The model under review builds one solid part; all positions refer to its coordinate system, in mm. A direction names the side the tool comes from. Coordinates: 2 decimals unless noted, no trailing zeros. Write each loop counter-clockwise with the first axis right and the second up, starting at its lowest first coordinate (ties: lowest second). Pieces come first, ordered by that corner, then holes. Notation, with made-up numbers: M 84,-39.5 L 102,-39.5 A17 cw 102,-20.5 Z; hole C 23,-36 d1. An arc over 180 degrees is marked long. Answer as CSV lines item,"result". Start each with the question number.
from build123d import *
from OCP.BRepFilletAPI import BRepFilletAPI_MakeChamfer

# Parameters (mm, degrees)
SKETCH_1_W          = 44.524667954
SKETCH_1_H          = 33.301696974
EXTRUDE_1_DEPTH     = 25
SKETCH_2_W          = 25
SKETCH_2_H          = 44.524667954
EXTRUDE_2_DEPTH     = 20
SKETCH_3_R          = 4
CUT_EXTRUDE_1_DEPTH = 67.802936569
SKETCH_4_W          = 57.585084074
SKETCH_4_H          = 20.16053609
CUT_EXTRUDE_2_DEPTH = 23
CHAMFER_2_SIZE      = 10
CHAMFER_2_SIZE2     = 6.494075932
SKETCH_5_W          = 25
SKETCH_5_H          = 60
EXTRUDE_3_DEPTH     = 12
FILLET_2_R          = 7
SKETCH_6_R          = 12.5
CUT_EXTRUDE_3_DEPTH = 59.13936943


with BuildPart() as part:
    # Эскиз1 → Вытянуть1 (new body)
    with BuildSketch(Plane(origin=(0, 0, 0), x_dir=(0, 0, -1), z_dir=(1, 0, 0))):
        with Locations((0, 6.421024908)):
            Rectangle(SKETCH_1_W, SKETCH_1_H)
    extrude(amount=EXTRUDE_1_DEPTH)

    # Эскиз2 → Вытянуть2 (add)
    with BuildSketch(Plane(origin=(0, 23.071873395, 0), x_dir=(1, 0, 0), z_dir=(0, 1, 0))):
        with Locations((12.5, 0)):
            Rectangle(SKETCH_2_W, SKETCH_2_H)
    extrude(amount=EXTRUDE_2_DEPTH)

    # Эскиз3 → Вырез-Вытянуть1 (cut, through all)
    with BuildSketch(Plane.XY.offset(22.262333977)):
        with Locations((12.457612309, 32.292854615)):
            Circle(SKETCH_3_R)
    extrude(amount=-CUT_EXTRUDE_1_DEPTH, mode=Mode.SUBTRACT)

    # Эскиз4 → Вырез-Вытянуть2 (cut)
    with BuildSketch(Plane(origin=(0, 43.071873395, 0), x_dir=(1, 0, 0), z_dir=(0, 1, 0))):
        Rectangle(SKETCH_4_W, SKETCH_4_H)
    extrude(amount=-CUT_EXTRUDE_2_DEPTH, mode=Mode.SUBTRACT)

    # Фаска2: one chamfer whose edges measure the first distance from different faces: ONE call of the kernel's chamfer builder (chamfer() names one face for all edges)
    chamfer_2_edges_1 = [part.edges().sort_by_distance(p)[0] for p in [
        (0, 43.071873395, -16.171301011),
        (0, 43.071873395, 16.171301011),
    ]]
    chamfer_2_side_1 = [part.faces().sort_by_distance(p)[0] for p in [
        (0, 12.741969901, 0),
    ]]
    chamfer_2_edges_2 = [part.edges().sort_by_distance(p)[0] for p in [
        (25, 43.071873395, 16.171301011),
        (25, 43.071873395, -16.171301011),
    ]]
    chamfer_2_side_2 = [part.faces().sort_by_distance(p)[0] for p in [
        (25, 12.741969901, 0),
    ]]
    chamfer_2 = BRepFilletAPI_MakeChamfer(part.part.solid().wrapped)
    for e in chamfer_2_edges_1:
        chamfer_2.Add(CHAMFER_2_SIZE, CHAMFER_2_SIZE2, e.wrapped, chamfer_2_side_1[0].wrapped)  # the first distance lies on this face
    for e in chamfer_2_edges_2:
        chamfer_2.Add(CHAMFER_2_SIZE, CHAMFER_2_SIZE2, e.wrapped, chamfer_2_side_2[0].wrapped)  # the first distance lies on this face
    add(Compound.cast(chamfer_2.Shape()), mode=Mode.REPLACE)

    # Эскиз5 → Вытянуть3 (add)
    with BuildSketch(Plane.XZ.offset(10.229823579)):
        with Locations((12.5, 0)):
            Rectangle(SKETCH_5_W, SKETCH_5_H)
    extrude(amount=EXTRUDE_3_DEPTH)

    # Скругление2
    fillet_2_edges = [part.edges().sort_by_distance(p)[0] for p in [
        (12.5, -10.229823579, -22.262333977),
        (12.5, -10.229823579, 22.262333977),
    ]]
    fillet(fillet_2_edges, radius=FILLET_2_R)

    # Эскиз6 → Вырез-Вытянуть3 (cut, through all)
    with BuildSketch(Plane(origin=(25, 0, 0), x_dir=(0, 0, -1), z_dir=(1, 0, 0))):
        with Locations((1.8e-08, 3.6e-08)):
            Circle(SKETCH_6_R)
    extrude(amount=-CUT_EXTRUDE_3_DEPTH, mode=Mode.SUBTRACT)


solid = part.part
1) Take a section at A-A on y = 0. Give the boundary of the cut face in (x, z).
2) Take a section at B-B on z = 0. Give the boundary of the cut face in (x, y).
3) To check wall thickness, follow line 1 (Y direction, x = 14.25, z = 0); line 2 (Z direction, x = 12.5, y = 38); line 3 (Y direction, x = 15.25, z = -11). State the ranges of each line that lie inside material, in increasing order. Write a range as [from, to].
4) Mouldability with a two-part tool opening along Z and no side actions: class faces 4 (the cylindrical face through (12.675, 3.755, -11.923)), 5 (the cylindrical face through (12.675, -8.234, 24.367)), 6 (the flat face through (12, 43.072, 16)) as +Z half, -Z half, draft (parallel to the pull), parting line (faces both ways), or undercut.
5) Tool access review of faces 1 (the flat face through (12, 20.072, 0)), 2 (the flat face through (12, 20, -22.262)), 3 (the flat face through (21.71, 38.14, -16.09)): name each direction out of +Z, -Z, +X, -X, +Y, -Y from which nothing blocks a thin tool from reaching the whole face with its end or side.
6) Take a section at C-C on x = 15.5. Give the boundary of the cut face in (y, z), and give its area (3 significant figures).
7) Clearance check with flat-ended pins moving along their axes: pin 1 Ø9 at (x, y) = (12.46, 32.29) entering from -Z; pin 2 Ø2 at (x, z) = (17.5, 0) entering from +Y; pin 3 Ø0.8 at (x, z) = (18, 29.5) entering from +Y; pin 4 Ø1.5 at (y, z) = (6, 9) entering from -X. State where each tip first meets the part, or that it passes through.
Results:
1,outline,"M 0,-22.26 L 25,-22.26 L 25,-12.5 L 0,-12.5 Z; M 0,12.5 L 25,12.5 L 25,22.26 L 0,22.26 Z"
2,outline,"M 0,-22.23 L 25,-22.23 L 25,-12.5 L 0,-12.5 Z; M 0,12.5 L 25,12.5 L 25,20.07 L 0,20.07 Z"
3,line 1,"y = [-22.23, -12.5], [12.5, 20.07]"
3,line 2,"z = [-22.26, -10.08], [10.08, 22.26]"
3,line 3,"y = [-22.23, -5.94], [5.94, 29.43], [35.16, 43.07]"
4,face 4,"undercut"
4,face 5,"+Z half"
4,face 6,"draft"
5,face 1,"+X, -X, +Y"
5,face 2,"-Z, +X, -X, +Y"
5,face 3,"+Z, -Z, +X, +Y"
6,outline,"M -22.23,-30 L -10.23,-30 L -10.23,-29.26 A7 cw -3.23,-22.26 L 29.7,-22.26 L 29.7,-10.08 L 20.07,-10.08 L 20.07,10.08 L 29.7,10.08 L 29.7,22.26 L -3.23,22.26 A7 cw -10.23,29.26 L -10.23,30 L -22.23,30 Z; M 34.89,-22.26 L 43.07,-22.26 L 43.07,-10.08 L 34.89,-10.08 Z; M 34.89,10.08 L 43.07,10.08 L 43.07,22.26 L 34.89,22.26 Z; hole C 0,0 d25"
6,area,"2,030 mm²"
7,pin 1,"stops at z = -22.26"
7,pin 2,"stops at y = 20.07"
7,pin 3,"stops at y = -10.23"
7,pin 4,"passes through"
